Geometry check sheet. Reference: the model listing, model coordinates, mm. Round coordinates to 2 decimals unless told otherwise and drop trailing zeros. Loops run counter-clockwise (first coordinate to the right, second up) from the corner with the lowest first, then second, coordinate; pieces in that order, holes last. Notation, with made-up numbers: M 71,65 L 87,65 A8 cw 87,70 Z; hole C 44,5.5 d1. An arc over 180 degrees is marked long. Use one line per item in the form item = value. Start each with the question number.
1. Material ranges on line 1 (X direction, y = 11, z = -4); line 2 (Z direction, x = -0.45, y = 1.25); line 3 (Z direction, x = -1.25, y = 3.75), recorded low to high.
2. Cross-section at D-D (x = -1.05). Record the boundary of the cut face in (y, z), then the cut area to 3 significant figures.
3. Draft check along X on faces 1 (the cylindrical face through (-2.303, -3.755, 11.923)), 2 (the flat face through (2.1, 9.2, 7.35)), 3 (the flat face through (-2.1, 7.35, -9.2)), 4 (the flat face through (-2.5, 8, 0)). Enter one of: pulls with the +X half, pulls with the -X half, needs draft (parallel to the pull), parting line crosses it, or undercut.
4. Go/stop test with a flat-tipped pin: pin 1 (1 mm diameter, centred on x = 0.5, y = 8.5, fed in from -Z). Record where the tip stops, or that it passes through.
5. Cross-section at A-A (z = 0). Record the boundary of the cut face in (x, y).
6. Cross-section at C-C (x = 1.35). Record the boundary of the cut face in (y, z).
```python
from build123d import *


with BuildPart() as part:
    # Sketch1 → Revolve1 (revolve)
    with BuildSketch(Plane.XY, mode=Mode.PRIVATE) as revolve1_sk:
        with BuildLine():
            Line((-2.5, 7.5), (-0.2, 7.5))
            Line((-0.2, 7.5), (0, 7.846410162))
            Line((0, 7.846410162), (0.2, 7.5))
            Line((0.2, 7.5), (2.5, 7.5))
            Line((2.5, 7.5), (2.5, 12.5))
            Line((2.5, 12.5), (2.1, 12.5))
            Line((2.1, 12.5), (2.1, 11.6))
            ThreePointArc((2.1, 11.6), (0, 9.5), (-2.1, 11.6))
            Line((-2.1, 11.6), (-2.1, 12.5))
            Line((-2.1, 12.5), (-2.5, 12.5))
            Line((-2.5, 12.5), (-2.5, 7.5))
        make_face()
    revolve(revolve1_sk.sketch.rotate(Axis((-2.5, 0, 0), (1, 0, 0)), 90), axis=Axis((-2.5, 0, 0), (1, 0, 0)))


solid = part.part
```
Reported:
q1.line_1 = -2.5 to -2.1, 2.1 to 2.5
q1.line_2 = -9.47 to -7.4, 7.4 to 9.47
q1.line_3 = -9.18 to -6.5, 6.5 to 9.18
q2.outline = C 0,0 d19.56; hole C 0,0 d15
q2.area = 124 mm²
q3.face_1 = needs draft
q3.face_2 = undercut
q3.face_3 = undercut
q3.face_4 = pulls with the -X half
q4.pin_1 = -5.28
q5.outline = M -2.5,-12.5 L -2.1,-12.5 L -2.1,-11.6 A2.1 cw 2.1,-11.6 L 2.1,-12.5 L 2.5,-12.5 L 2.5,-7.5 L 0.2,-7.5 L 0,-7.85 L -0.2,-7.5 L -2.5,-7.5 Z; M -2.5,7.5 L -0.2,7.5 L 0,7.85 L 0.2,7.5 L 2.5,7.5 L 2.5,12.5 L 2.1,12.5 L 2.1,11.6 A2.1 cw -2.1,11.6 L -2.1,12.5 L -2.5,12.5 Z
q6.outline = C 0,0 d19.98; hole C 0,0 d15
